from build123d import *

# Parameters (mm, degrees)
SKETCH_1_R      = 1.55
EXTRUDE_1_DEPTH = 5.5


with BuildPart() as part:
    # ｽｹｯﾁ1 → ﾎﾞｽ - 押し出し1 (new body)
    with BuildSketch(Plane(origin=(0, 0, 0), x_dir=(1, 0, 0), z_dir=(0, 1, 0))):
        with BuildLine():
            Line((-7.985272428, -18.616517506), (-4.985272428, 20.383482494))
            ThreePointArc((-4.985272428, 20.383482494), (-1.734731239, 24.689425075), (3.535533906, 23.535533906))
            Line((3.535533906, 23.535533906), (23.535533906, 3.535533906))
            ThreePointArc((23.535533906, 3.535533906), (24.994366167, -0.237290102), (23.184407235, -3.854808758))
            Line((23.184407235, -3.854808758), (0.184407235, -22.854808758))
            ThreePointArc((0.184407235, -22.854808758), (-5.302511031, -23.438292797), (-7.985272428, -18.616517506))
        make_face()
        with Locations(Location((0, 20, 0), (0, 0, 270))):
            Circle(SKETCH_1_R, mode=Mode.SUBTRACT)
        with Locations(Location((0, 0, 0), (0, 0, 270))):
            Circle(SKETCH_1_R, mode=Mode.SUBTRACT)
        with Locations(Location((20, 0, 0), (0, 0, 270))):
            Circle(SKETCH_1_R, mode=Mode.SUBTRACT)
        with Locations(Location((-3, -19, 0), (0, 0, 270))):
            Circle(SKETCH_1_R, mode=Mode.SUBTRACT)
    extrude(amount=EXTRUDE_1_DEPTH)


solid = part.part
Verification items for the finished model (mm, model axes). Give positions to 0.01 mm unless a question says otherwise; leave off trailing zeros. Loops run counter-clockwise (first coordinate to the right, second up) from the corner with the lowest first, then second, coordinate; pieces in that order, holes last.
1) Thickness scan on line 1 along X through (y, z) = (1.6, 0); line 2 along X through (y, z) = (2.2, 19); line 3 along X through (y, z) = (3.6, -20). Record the ranges inside material, lowest first.
2) Draft check along Z on faces 1 (the flat face through (11.85, 2.71, 13.22)), 2 (the flat face through (-6.506, 2.712, -0.61)), 3 (the cylindrical face through (0.466, 2.712, 1.478)). Enter one of: pulls with the +Z half, pulls with the -Z half, needs draft (parallel to the pull), parting line crosses it, or undercut.
3) Sectioned sample at A-A, the plane x = 20. Enter the section's corners in (y, z).
4) Sectioned sample at D-D, the plane x = -0.5. Enter the section's corners in (y, z), then the cut area to 3 significant figures.
5) Sectioned sample at C-C, the plane y = 0.9. Enter the section's corners in (x, z).
6) Depth check by flat-ended pin: pin 1 Ø3 at (y, z) = (2, 7.5) entering from -X; pin 2 Ø2 at (y, z) = (3.5, 5.5) entering from +X. Enter the tip coordinate at first touch or a pass-through.
7) Sectioned sample at B-B, the plane z = 20. Enter the section's corners in (x, y), then the cut area to 3 significant figures.
Answers:
1. line 1: x = -6.55 to -1.55, 1.55 to 18.45, 21.55 to 25
1. line 2: x = -8 to -4.55, -1.45 to 4.85
1. line 3: x = -5.01 to -1.55, 1.55 to 7.07
2. face 1: pulls with the +Z half
2. face 2: pulls with the -Z half
2. face 3: undercut
3. outline: (0, -7.07) - (5.5, -7.07) - (5.5, -1.55) - (0, -1.55) - close; (0, 1.55) - (5.5, 1.55) - (5.5, 6.49) - (0, 6.49) - close
4. outline: (0, -24.97) - (5.5, -24.97) - (5.5, -21.47) - (0, -21.47) - close; (0, -18.53) - (5.5, -18.53) - (5.5, -1.47) - (0, -1.47) - close; (0, 1.47) - (5.5, 1.47) - (5.5, 23.33) - (0, 23.33) - close
4. area: 233 mm2
5. outline: (-7.99, 18.62) - (-4.99, -20.38) arc R5 ccw to (3.54, -23.54) - (23.54, -3.54) arc R5 ccw to (23.18, 3.85) - (0.18, 22.85) arc R5 ccw to start; hole circle Ø3.1 at (-3, 19); hole circle Ø3.1 at (0, -20); hole circle Ø3.1 at (0, 0); hole circle Ø3.1 at (20, 0)
6. pin 1: stops at x = -7.25
6. pin 2: stops at x = 22.4
7. outline: (-7.9, 0) - (-4.18, 0) - (-4.18, 5.5) - (-7.9, 5.5) - close; (-1.82, 0) - (3.64, 0) - (3.64, 5.5) - (-1.82, 5.5) - close
7. area: 50.4 mm2
